Verification items for the finished model (mm, model axes). A direction names the side the tool comes from. Give positions to 0.01 mm unless a question says otherwise; leave off trailing zeros. Loops run counter-clockwise (first coordinate to the right, second up) from the corner with the lowest first, then second, coordinate; pieces in that order, holes last. Notation, with made-up numbers: M 5.5,13 L 44.5,13 A13 ccw 44.5,18 Z; hole C 16,25 d2. An arc over 180 degrees is marked long. Answer in a Markdown table with one row per item.
```python
from build123d import *

# Parameters (mm, degrees)
F0_W          = 127.2562742233
F0_H          = 50.8075356483
F1_DEPTH      = 63.5
F1_DEPTH_BACK = 63.5
F3_DEPTH      = 12.7
F4_R          = 12.69999
F5_W          = 16.97918742
F5_H          = 25.4037678242
F6_DEPTH      = 31.75


# Not quite as in the source:
# - a fillet or chamfer is up to 0.001 mm smaller than in the source, because OpenCascade refuses the exact size


with BuildPart() as f1:
    # F0 (on Front) → F1 (new body, two sides)
    with BuildSketch(Plane.XZ) as f1_sk:
        with Locations((0, 25.4037678242)):
            Rectangle(F0_W, F0_H)
    extrude(amount=F1_DEPTH)
    extrude(f1_sk.sketch, amount=-F1_DEPTH_BACK)

    # F2 (on face) → F3 (cut)
    with BuildSketch(Plane.XY.offset(50.8075356483)):
        Polygon((0, -25.4037678242), (0, 0), (0, 25.4037678242), (-42.37918742, 25.4037678242), (-42.37918742, 0), (-42.37918742, -25.4037678242), align=None)
    extrude(amount=-F3_DEPTH, mode=Mode.SUBTRACT)

    # F4 (radius 12.7 in the source; OpenCascade refuses exactly that, so slightly less here)
    f4_edges = [f1.edges().sort_by_distance(p)[0] for p in [
        (-42.379187, 0, 38.107536),
        (0, 0, 38.107536),
    ]]
    fillet(f4_edges, radius=F4_R)

    # F5 (on face) → F6 (join)
    with BuildSketch(Plane.XY.offset(38.1075356483)):
        with Locations((-21.18959371, -0.1187091693)):
            Rectangle(F5_W, F5_H)
    extrude(amount=F6_DEPTH)


solid = f1.part
```
Item 1: Sectioned sample at A-A (x = -25). Record the cut outline in (y, z).
Reported:
| item | result |
|---|---|
| outline | M -63.5,0 L 63.5,0 L 63.5,50.81 L 25.4,50.81 L 25.4,38.11 L 12.58,38.11 L 12.58,69.86 L -12.82,69.86 L -12.82,38.11 L -25.4,38.11 L -25.4,50.81 L -63.5,50.81 Z |
Item 2: Go/stop test with a flat-tipped pin: pin 1 (12 mm diameter, centred on x = -41, y = 3.5, fed in from +Z). Record where the tip stops, or that it passes through.
Reported:
| item | result |
|---|---|
| pin 1 | stops at z = 50.81 |
Item 3: Scan lines: L1, parallel to Y at x = -28, z = 38.5; L2, parallel to Z at x = 31, y = 21; L3, parallel to Z at x = -20, y = -16.5. Record each from-to range of solid material in increasing order. Write a range as [from, to].
Reported:
| item | result |
|---|---|
| L1 | y = [-63.5, -25.4], [-12.82, 12.58], [25.4, 63.5] |
| L2 | z = [0, 50.81] |
| L3 | z = [0, 38.11] |
Item 4: Release check for a two-part mould opening along Y. For faces 3 (the flat face through (13, -1, 50.808)), 4 (the flat face through (-1, -63.5, 26)), 5 (the flat face through (-21, 17, 38.108)), 6 (the flat face through (-29.679, 0, 54)) record: released by +Y, released by -Y, zero draft, split by the parting line, or undercut.
Reported:
| item | result |
|---|---|
| face 3 | zero draft |
| face 4 | released by -Y |
| face 5 | undercut |
| face 6 | undercut |
Item 5: Sectioned sample at C-C (z = 63). Record the cut outline in (x, y), and give its area (3 significant figures).
Reported:
| item | result |
|---|---|
| outline | M -29.68,-12.82 L -12.7,-12.82 L -12.7,12.58 L -29.68,12.58 Z |
| area | 431 mm^2 |
Item 6: Tool access check on faces 1 (the flat face through (-1, 63.5, 26)), 2 (the cylindrical face through (-38.76, -0.36, 41.93)). Record the directions out of +Z, -Z, +X, -X, +Y, -Y that give a thin tool (end or side, any length) a straight path to the whole face; none if there is none.
Reported:
| item | result |
|---|---|
| face 1 | +Z, -Z, +X, -X, +Y |
| face 2 | +Z |
